CAD build for the part. Positions are in the model's coordinates, mm. A direction names the side the tool comes from. Give positions to 0.01 mm unless a question says otherwise; leave off trailing zeros. Write each loop counter-clockwise with the first axis right and the second up, starting at its lowest first coordinate (ties: lowest second). Pieces come first, ordered by that corner, then holes. Notation, with made-up numbers: (46.25, -37.75) -> (60.25, -37.75) arc R20 cw to (60.25, -0.75) -> close; hole circle Ø2 at (-21, 30). An arc over 180 degrees is marked (long way). Answer as a JSON object with one key per item and string values.
```python
from build123d import *

# Parameters (mm, degrees)
F0_R     = 29.9974
F0_R_2   = 8.001
F1_DEPTH = 10.16
F0_R_3   = 35.0012
F2_DEPTH = 15.0114
F3_DEPTH = 19.5072


with BuildPart() as f1:
    # F0 (on Front) → F1 (new body)
    with BuildSketch(Plane.XZ):
        Circle(F0_R)
        with BuildLine():
            ThreePointArc((8.001, -20.5599348992), (-5.6575613563, -26.2174962555), (0, -12.5589348992))
            ThreePointArc((0, -12.5589348992), (5.6575613563, -14.9023735429), (8.001, -20.5599348992))
        make_face(mode=Mode.SUBTRACT)
        with Locations((-20.5486, 0)):
            Circle(F0_R_2, mode=Mode.SUBTRACT)
        with BuildLine():
            ThreePointArc((0, 9.9949), (7.0674615673, 7.0674615673), (9.9949, 0))
            ThreePointArc((9.9949, 0), (7.0674615673, -7.0674615673), (0, -9.9949))
            ThreePointArc((0, -9.9949), (-9.9949, 0), (0, 9.9949))
        make_face(mode=Mode.SUBTRACT)
        with BuildLine():
            ThreePointArc((28.5496, 0), (20.5486, -8.001), (12.5476, 0))
            ThreePointArc((12.5476, 0), (20.5486, 8.001), (28.5496, 0))
        make_face(mode=Mode.SUBTRACT)
        with BuildLine():
            ThreePointArc((8.001, 20.5599348992), (5.6575613563, 14.9023735429), (0, 12.5589348992))
            ThreePointArc((0, 12.5589348992), (-5.6575613563, 26.2174962555), (8.001, 20.5599348992))
        make_face(mode=Mode.SUBTRACT)
    extrude(amount=F1_DEPTH)

    # F0 (on Front) → F2 (join)
    with BuildSketch(Plane.XZ):
        Circle(F0_R_3)
        Circle(F0_R, mode=Mode.SUBTRACT)
    extrude(amount=F2_DEPTH)

    # F0 (on Front) → F3 (join)
    with BuildSketch(Plane.XZ):
        with BuildLine():
            Line((9.9949, 0), (6.3373, 0))
            ThreePointArc((6.3373, 0), (4.4811478044, -4.4811478044), (0, -6.3373))
            Line((0, -6.3373), (0, -9.9949))
            ThreePointArc((0, -9.9949), (7.0674615673, -7.0674615673), (9.9949, 0))
        make_face()
        with BuildLine():
            ThreePointArc((0, 6.3373), (4.4811478044, 4.4811478044), (6.3373, 0))
            Line((6.3373, 0), (9.9949, 0))
            ThreePointArc((9.9949, 0), (7.0674615673, 7.0674615673), (0, 9.9949))
            Line((0, 9.9949), (0, 6.3373))
        make_face()
        with BuildLine():
            ThreePointArc((0, -6.3373), (-6.3373, 0), (0, 6.3373))
            Line((0, 6.3373), (0, 9.9949))
            ThreePointArc((0, 9.9949), (-9.9949, 0), (0, -9.9949))
            Line((0, -9.9949), (0, -6.3373))
        make_face()
    extrude(amount=F3_DEPTH)


solid = f1.part
```
1) 3-axis set-ups, long thin cutter, end or side, ignore diameter. For faces 1 (the cylindrical face through (-29.97, -12.55, 1.32)), 2 (the cylindrical face through (-12.917, -5.009, 2.403)): which of +Z, -Z, +X, -X, +Y, -Y reach the whole face in a straight line?
Model answer:
{"face 1": "-Y", "face 2": "+Y, -Y"}
2) Mould opens along Z. For faces 3 (the flat face through (7, -19.507, 0)), 4 (the flat face through (13, -10.16, -6)), 5 (the cylindrical face through (33.385, -7.401, 10.513)) say: released by +Z, released by -Z, zero draft, split by the parting line, or undercut.
Model answer:
{"face 3": "zero draft", "face 4": "undercut", "face 5": "split by the parting line"}
3) Slice it at D-D (x = 19.5). List the corners of the cut face in (y, z).
Model answer:
{"outline": "(-15.01, -29.07) -> (0, -29.07) -> (0, -7.93) -> (-10.16, -7.93) -> (-10.16, -22.79) -> (-15.01, -22.79) -> close; (-15.01, 22.79) -> (-10.16, 22.79) -> (-10.16, 7.93) -> (0, 7.93) -> (0, 29.07) -> (-15.01, 29.07) -> close"}
4) Slice it at A-A (y = -11.5). List the corners of the cut face in (x, z).
Model answer:
{"outline": "circle Ø70 at (0, 0); circle Ø19.99 at (0, 0); hole circle Ø59.99 at (0, 0); hole circle Ø12.67 at (0, 0)"}
5) Pin check, flat tips, straight feed: pin 1 (5 mm diameter, centred on y = -15, z = 15, fed in from -X); pin 2 (1.5 mm diameter, centred on x = 5.5, z = 24, fed in from +Y); pin 3 (10 mm diameter, centred on x = -13, y = -12, fed in from +Z); pin 4 (5 mm diameter, centred on y = -9.5, z = 16, fed in from +X). Stop position of each tip, or through.
Model answer:
{"pin 1": "stops at x = -32.69", "pin 2": "passes through", "pin 3": "stops at z = 34.07", "pin 4": "stops at x = 32.29"}
6) Wall check: probe 1 along Y at (x, z) = (25.5, 14); probe 2 along Y at (x, z) = (30, -11.5); probe 3 along Z at (x, y) = (5.5, -11.5). Give the ranges that are in metal, low to high.
Model answer:
{"probe 1": "y = -10.16 to 0", "probe 2": "y = -15.01 to 0", "probe 3": "z = -34.57 to -29.49, -8.35 to -3.15, 3.15 to 8.35, 29.49 to 34.57"}
7) Slice it at B-B (y = -5.25). List the corners of the cut face in (x, z).
Model answer:
{"outline": "circle Ø70 at (0, 0); hole circle Ø16 at (-20.55, 0); hole circle Ø16 at (0, -20.56); hole circle Ø16 at (0, 20.56); hole circle Ø12.67 at (0, 0); hole circle Ø16 at (20.55, 0)"}
8) Slice it at C-C (z = 26). List the corners of the cut face in (x, y), then the cut area to 3 significant figures.
Model answer:
{"outline": "(-23.43, -15.01) -> (-14.96, -15.01) -> (-14.96, -10.16) -> (-5.87, -10.16) -> (-5.87, 0) -> (-23.43, 0) -> close; (5.87, -10.16) -> (14.96, -10.16) -> (14.96, -15.01) -> (23.43, -15.01) -> (23.43, 0) -> (5.87, 0) -> close", "area": "439 mm2"}
